For this review, use the dimensioned drawing (mm, ordinates from the lowest corner) and the shaded views. A direction names the side the tool comes from. Round coordinates to 2 decimals unless told otherwise and drop trailing zeros. Loops run counter-clockwise (first coordinate to the right, second up) from the corner with the lowest first, then second, coordinate; pieces in that order, holes last. Notation, with made-up numbers: M -14,-11 L 27,-11 A18 ccw 27,6 Z; hole C -11.5,64 d10. An arc over 180 degrees is marked long. One line per item, written item: value. Start each with the question number.
Item 1: We need section A-A (x = 3). Write out the cut boundary in (y, z), then the cut area to 3 significant figures.
Item 2: Mouldability with a two-part tool opening along X and no side actions: class the marked faces 1, 2, 3 and 4 as released by +X, released by -X, zero draft, split by the parting line, or undercut.
Item 3: We need section B-B (z = 3). Write out the cut boundary in (x, y), then the cut area to 3 significant figures.
Item 4: We need section C-C (y = 4.5). Write out the cut boundary in (x, z), then the cut area to 3 significant figures.
Item 5: For the marked faces 5, 6, 7, 8 and 9, list the 3-axis set-ups (+Z, -Z, +X, -X, +Y, -Y) from which the entire face can be reached by the end or side of a thin tool; tool diameter is ignored.
Item 6: We need section D-D (x = 35.5). Write out the cut boundary in (y, z), then the cut area to 3 significant figures.
Item 7: Clearance check with flat-ended pins moving along their axes: pin 1 (1.5 mm diameter, centred on x = 4.5, y = 2, fed in from -Z); pin 2 (3 mm diameter, centred on x = 20.5, z = 25, fed in from +Y); pin 3 (3 mm diameter, centred on x = 32.5, y = 4.5, fed in from +Z); pin 4 (1.5 mm diameter, centred on x = 19, y = 2.5, fed in from +Z). State where each tip first meets the part, or that it passes through.
Item 8: For line 1 along X through (y, z) = (0.85, 29); line 2 along Z through (x, y) = (39, 1.25); line 3 along Y through (x, z) = (21.5, 30.5), list the stretches that pass through material, from the lowest coordinate up.
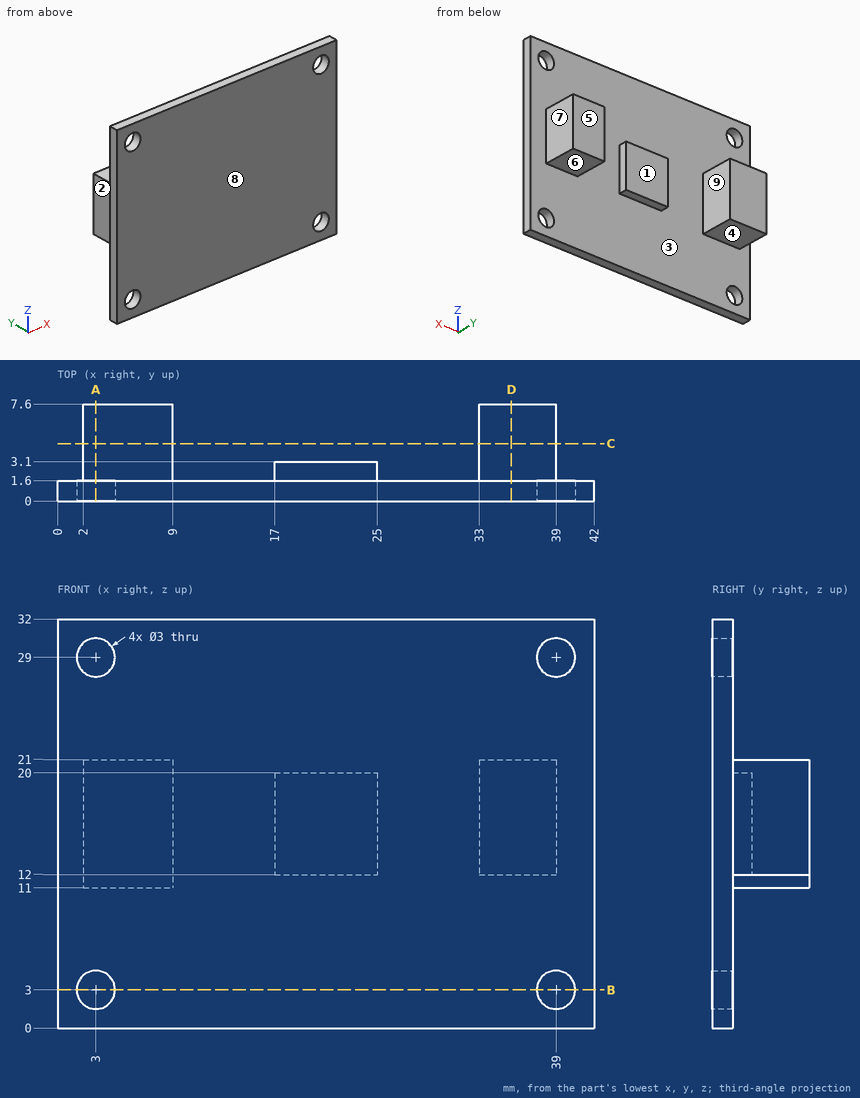
A:
1. outline: M 0,0 L 1.6,0 L 1.6,1.5 L 0,1.5 Z; M 0,4.5 L 1.6,4.5 L 1.6,11 L 7.6,11 L 7.6,21 L 1.6,21 L 1.6,27.5 L 0,27.5 Z; M 0,30.5 L 1.6,30.5 L 1.6,32 L 0,32 Z
1. area: 102 mm2
2. face 1: undercut
2. face 2: released by -X
2. face 3: undercut
2. face 4: zero draft
3. outline: M 0,0 L 1.5,0 L 1.5,1.6 L 0,1.6 Z; M 4.5,0 L 37.5,0 L 37.5,1.6 L 4.5,1.6 Z; M 40.5,0 L 42,0 L 42,1.6 L 40.5,1.6 Z
3. area: 57.6 mm2
4. outline: M 2,11 L 9,11 L 9,21 L 2,21 Z; M 33,12 L 39,12 L 39,21 L 33,21 Z
4. area: 124 mm2
5. face 5: +Z, -Z, +X, -X, +Y
5. face 6: -Z, +X, +Y
5. face 7: +Z, -Z, +X, +Y
5. face 8: +Z, -Z, +X, -X, -Y
5. face 9: +Z, -Z, +Y
6. outline: M 0,0 L 1.6,0 L 1.6,12 L 7.6,12 L 7.6,21 L 1.6,21 L 1.6,32 L 0,32 Z
6. area: 105 mm2
7. pin 1: z = 0
7. pin 2: y = 1.6
7. pin 3: z = 21
7. pin 4: z = 20
8. line 1: 0 to 1.5, 4.5 to 37.5, 40.5 to 42
8. line 2: 0 to 1.5, 4.5 to 27.5, 30.5 to 32
8. line 3: 0 to 1.6
